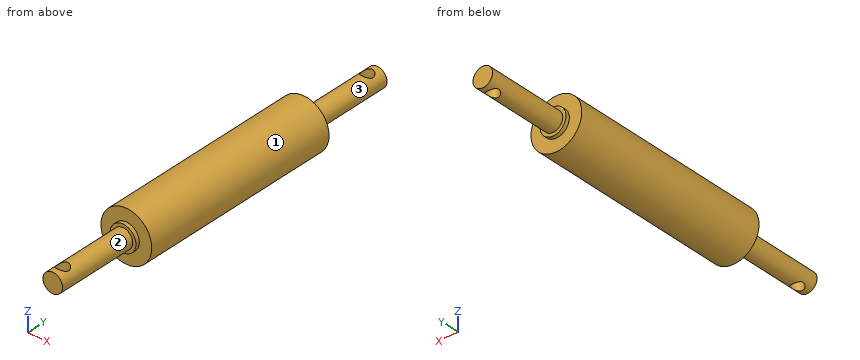
from build123d import *

# Parameters (mm, degrees)
SKETCH1_R                = 13
BOSS_EXTRUDE1_DEPTH      = 53
BOSS_EXTRUDE1_DEPTH_BACK = 53
SKETCH2_R                = 6.65
BOSS_EXTRUDE2_DEPTH      = 2
SKETCH3_R                = 5
BOSS_EXTRUDE3_DEPTH      = 42
SKETCH4_R                = 3.05
CUT_EXTRUDE1_DEPTH       = 14


with BuildPart() as part:
    # Sketch1 → Boss-Extrude1 (new body, two sides)
    with BuildSketch(Plane(origin=(0, 0, 0), x_dir=(1, 0, 0), z_dir=(0, 1, 0))) as boss_extrude1_sk:
        Circle(SKETCH1_R)
    extrude(amount=BOSS_EXTRUDE1_DEPTH)
    extrude(boss_extrude1_sk.sketch, amount=-BOSS_EXTRUDE1_DEPTH_BACK)

    # Sketch2 → Boss-Extrude2 (add)
    with BuildSketch(Plane(origin=(0, 53, 0), x_dir=(1, 0, 0), z_dir=(0, 1, 0))):
        Circle(SKETCH2_R)
    boss_extrude2 = extrude(amount=BOSS_EXTRUDE2_DEPTH)

    # Sketch3 → Boss-Extrude3 (add)
    with BuildSketch(Plane(origin=(0, 55, 0), x_dir=(1, 0, 0), z_dir=(0, 1, 0))):
        Circle(SKETCH3_R)
    boss_extrude3 = extrude(amount=BOSS_EXTRUDE3_DEPTH)

    # Mirror1: Boss-Extrude2, Boss-Extrude3 across plane
    add(boss_extrude2.mirror(Plane.ZX))
    add(boss_extrude3.mirror(Plane.ZX))

    # Sketch4 → Cut-Extrude1 (cut, symmetric)
    with BuildSketch(Plane.XY):
        with Locations((0, 91)):
            Circle(SKETCH4_R)
    cut_extrude1 = extrude(amount=CUT_EXTRUDE1_DEPTH, both=True, mode=Mode.SUBTRACT)

    # Mirror2: Cut-Extrude1 across plane
    add(cut_extrude1.mirror(Plane.ZX), mode=Mode.SUBTRACT)


solid = part.part
The listing builds one solid part. Answer for the finished solid, in the listing's coordinates (mm). Face numbers are marked on the shaded views. A direction names the side the tool comes from. Give positions to 0.01 mm unless a question says otherwise; leave off trailing zeros. Order: outer loops, then holes, each group sorted by start corner. A loop starts at its lowest first (then second) coordinate and runs counter-clockwise, first axis right, second up. Notation, with made-up numbers: (15.5, -17.75) - (59.5, -17.75) arc R27 ccw to (59.5, 17.25) - close; hole circle Ø4 at (84.25, 71.25). An arc over 180 degrees is marked (long way). Answer as CSV lines item,"result".
Q1. A cutting plane is placed at C-C, the plane y = -60. Determine the outline of the cut face in (x, z).
Answer key:
outline,"circle Ø10 at (0, 0)"
Q2. Straight lines are drawn through the part: L1, parallel to Y at x = 0, z = 0.5; L2, parallel to X at y = -91, z = -0.5; L3, parallel to Y at x = 1.75, z = 4. For each, find the intervals that lie inside material, in ascending order.
Answer key:
L1,"y = -97 to -94.05, -87.95 to 87.95, 94.05 to 97"
L2,"x = -4.97 to -3.05, 3.05 to 4.97"
L3,"y = -97 to -93.5, -88.5 to 88.5, 93.5 to 97"
Q3. A cutting plane is placed at B-B, the plane z = 0. Determine the outline of the cut face in (x, y).
Answer key:
outline,"(-13, -53) - (-6.65, -53) - (-6.65, -55) - (-5, -55) - (-5, -97) - (5, -97) - (5, -55) - (6.65, -55) - (6.65, -53) - (13, -53) - (13, 53) - (6.65, 53) - (6.65, 55) - (5, 55) - (5, 97) - (-5, 97) - (-5, 55) - (-6.65, 55) - (-6.65, 53) - (-13, 53) - close; hole circle Ø6.1 at (0, -91); hole circle Ø6.1 at (0, 91)"
Q4. A cutting plane is placed at D-D, the plane y = -91. Determine the outline of the cut face in (x, z), and give its area (3 significant figures).
Answer key:
outline,"(-3.05, -3.96) - (-3.05, 3.96) arc R5 ccw to start; (3.05, -3.96) arc R5 ccw to (3.05, 3.96) - close"
area,"21.6 mm^2"
Q5. Which of the six approach directions +Z, -Z, +X, -X, +Y, -Y give full straight-line access (tool end or side, diameter ignored) to the marked faces 1, 2 and 3?
Answer key:
face 1,"+Y, -Y"
face 2,"-Y"
face 3,"+Y"
Q6. Each of these flat-tipped pins is pushed along its axis until it touches: pin 1 Ø5 at (y, z) = (-60, -3.5) entering from +X; pin 2 Ø7 at (x, y) = (0, 91) entering from +Z; pin 3 Ø3 at (x, z) = (-1, -9.5) entering from +Y. Where does it stop, or does it pass through?
Answer key:
pin 1,"stops at x = 4.9"
pin 2,"stops at z = 5"
pin 3,"stops at y = 53"
Q7. A cutting plane is placed at A-A, the plane x = 0. Determine the outline of the cut face in (y, z).
Answer key:
outline,"(-97, -5) - (-94.05, -5) - (-94.05, 5) - (-97, 5) - close; (-87.95, -5) - (-55, -5) - (-55, -6.65) - (-53, -6.65) - (-53, -13) - (53, -13) - (53, -6.65) - (55, -6.65) - (55, -5) - (87.95, -5) - (87.95, 5) - (55, 5) - (55, 6.65) - (53, 6.65) - (53, 13) - (-53, 13) - (-53, 6.65) - (-55, 6.65) - (-55, 5) - (-87.95, 5) - close; (94.05, -5) - (97, -5) - (97, 5) - (94.05, 5) - close"
